Input: part model. Units: mm. Frame: model coordinates. A direction names the side the tool comes from. Coordinates: 2 decimals unless noted, no trailing zeros. Loops run counter-clockwise (first coordinate to the right, second up) from the corner with the lowest first, then second, coordinate; pieces in that order, holes last.
(1) Line query: L1, parallel to Y at x = 0, z = 14; L2, parallel to X at y = -14.5, z = 26; L3, parallel to Y at x = -5.5, z = 5. Output: solid intervals per line, ascending.
(2) Mould query, pull axis Y, two halves, no side actions, for faces 1 (the face through (15.785, 4.971, 21.571)), 2 (the face through (-18.953, 0.834, 41.281)), 3 (the face through (0, 0, 4.572)), 4 (the face through (0, 0, 0)). Classes: released by +Y, released by -Y, zero draft, split by the parting line, or undercut.
(3) Set-up query: faces 5 (the face through (0, 0, 38.1)), 6 (the face through (-2.579, 19.643, 18.783)). Return all of +Z, -Z, +X, -X, +Y, -Y with unobstructed straight access to the full face (end or side cutting, diameter ignored); none if empty.
(4) Contact query for flat-ended pins moving along their axis: P1, Ø5, axis at x = -3.5, y = -10.5, coming from the +Z side; P2, Ø4, axis at y = -11.5, z = 55.5, coming from the -X side; P3, Ø16.5, axis at x = 6.5, y = -3, coming from the -Z side; P4, Ø4, axis at x = -9.5, z = 34, coming from the -Y side. Output: stop coordinate, or through.
(5) Section A-A, the plane z = 24.5. Return loops of the section in (x, y), then the cut area to 3 significant figures.
(6) Section B-B, the plane z = 39. Return loops of the section in (x, y).
```python
from build123d import *

# Parameters (mm, degrees)
F0_R     = 19.812
F1_DEPTH = 38.1
F2_R     = 16.548802
F3_DEPTH = 33.528
F4_R     = 18.971562
F5_DEPTH = 25.4
F6_R     = 18.9484


with BuildPart() as f1:
    # F0 (on Top) → F1 (new body)
    with BuildSketch(Plane.XY):
        Circle(F0_R)
    extrude(amount=F1_DEPTH)

    # F2 (on face) → F3 (cut)
    with BuildSketch(Plane.XY.offset(38.1)):
        Circle(F2_R)
    extrude(amount=-F3_DEPTH, mode=Mode.SUBTRACT)

    # F4 (on face) → F5 (join)
    with BuildSketch(Plane.XY.offset(38.1)):
        Circle(F4_R)
    extrude(amount=F5_DEPTH)

    # F6
    f6_edges = [f1.edges().sort_by_distance(p)[0] for p in [
        (-18.971562, 0, 63.5),
    ]]
    fillet(f6_edges, radius=F6_R)


solid = f1.part
```
Report:
1. L1: y = -19.81 to -16.55, 16.55 to 19.81
1. L2: x = -13.5 to -7.98, 7.98 to 13.5
1. L3: y = -19.03 to -15.61, 15.61 to 19.03
2. face 1: undercut
2. face 2: split by the parting line
2. face 3: undercut
2. face 4: zero draft
3. face 5: none
3. face 6: +Z, -Z
4. P1: stops at z = 61.46
4. P2: stops at x = -12.93
4. P3: stops at z = 0
4. P4: stops at y = -18.34
5. outline: circle Ø39.62 at (0, 0); hole circle Ø33.1 at (0, 0)
5. area: 373 mm2
6. outline: circle Ø37.94 at (0, 0)
